from build123d import *

# Parameters (mm, degrees)
SKETCH2_R           = 19
SKETCH2_R_2         = 1.3
BOSS_EXTRUDE1_DEPTH = 8
SKETCH3_R           = 30
SKETCH3_R_2         = 17.487995661
BOSS_EXTRUDE2_DEPTH = 8
SKETCH4_R           = 2.9
BOSS_EXTRUDE3_DEPTH = 2
SKETCH6_R           = 5
BOSS_EXTRUDE4_DEPTH = 3
SKETCH5_R           = 3
CUT_EXTRUDE1_DEPTH  = 3
SKETCH7_R           = 25
CUT_EXTRUDE2_DEPTH  = 8
FILLET2_R           = 5


with BuildPart() as part:
    # Sketch2 → Boss-Extrude1 (new body)
    with BuildSketch(Plane.XY.offset(10)):
        Circle(SKETCH2_R)
        with Locations((0, -2.215732779)):
            Circle(SKETCH2_R_2, mode=Mode.SUBTRACT)
        with Locations((3.9, -2.215732779)):
            Circle(SKETCH2_R_2, mode=Mode.SUBTRACT)
        with Locations((7.8, -2.215732779)):
            Circle(SKETCH2_R_2, mode=Mode.SUBTRACT)
        with Locations((11.7, -2.215732779)):
            Circle(SKETCH2_R_2, mode=Mode.SUBTRACT)
        with Locations((1.95, -5.593231854)):
            Circle(SKETCH2_R_2, mode=Mode.SUBTRACT)
        with Locations((3.9, -8.970730929)):
            Circle(SKETCH2_R_2, mode=Mode.SUBTRACT)
        with Locations((5.850000003, -12.348230002)):
            Circle(SKETCH2_R_2, mode=Mode.SUBTRACT)
        with Locations((-1.95, -5.593231854)):
            Circle(SKETCH2_R_2, mode=Mode.SUBTRACT)
        with Locations((-3.9, -8.970730929)):
            Circle(SKETCH2_R_2, mode=Mode.SUBTRACT)
        with Locations((-5.85, -12.348230004)):
            Circle(SKETCH2_R_2, mode=Mode.SUBTRACT)
        with Locations((-3.9, -2.215732779)):
            Circle(SKETCH2_R_2, mode=Mode.SUBTRACT)
        with Locations((-7.8, -2.215732779)):
            Circle(SKETCH2_R_2, mode=Mode.SUBTRACT)
        with Locations((-11.7, -2.215732779)):
            Circle(SKETCH2_R_2, mode=Mode.SUBTRACT)
        with Locations((-1.950000001, 1.161766295)):
            Circle(SKETCH2_R_2, mode=Mode.SUBTRACT)
        with Locations((-3.9, 4.53926537)):
            Circle(SKETCH2_R_2, mode=Mode.SUBTRACT)
        with Locations((-5.85, 7.916764445)):
            Circle(SKETCH2_R_2, mode=Mode.SUBTRACT)
        with Locations((-7.8, 11.29426352)):
            Circle(SKETCH2_R_2, mode=Mode.SUBTRACT)
        with Locations((1.95, 1.161766295)):
            Circle(SKETCH2_R_2, mode=Mode.SUBTRACT)
        with Locations((3.9, 4.53926537)):
            Circle(SKETCH2_R_2, mode=Mode.SUBTRACT)
        with Locations((5.85, 7.916764445)):
            Circle(SKETCH2_R_2, mode=Mode.SUBTRACT)
        with Locations((7.8, 11.29426352)):
            Circle(SKETCH2_R_2, mode=Mode.SUBTRACT)
        with Locations((5.85, 1.161766295)):
            Circle(SKETCH2_R_2, mode=Mode.SUBTRACT)
        with Locations((7.8, 4.53926537)):
            Circle(SKETCH2_R_2, mode=Mode.SUBTRACT)
        with Locations((9.75, 1.161766295)):
            Circle(SKETCH2_R_2, mode=Mode.SUBTRACT)
        with Locations((11.7, 4.53926537)):
            Circle(SKETCH2_R_2, mode=Mode.SUBTRACT)
        with Locations((9.749099848, 7.918323553)):
            Circle(SKETCH2_R_2, mode=Mode.SUBTRACT)
        with Locations((13.650900152, 1.160207187)):
            Circle(SKETCH2_R_2, mode=Mode.SUBTRACT)
        with Locations((5.850000208, -5.594790783)):
            Circle(SKETCH2_R_2, mode=Mode.SUBTRACT)
        with Locations((9.750000208, -5.594790782)):
            Circle(SKETCH2_R_2, mode=Mode.SUBTRACT)
        with Locations((7.800000209, -8.972289857)):
            Circle(SKETCH2_R_2, mode=Mode.SUBTRACT)
        with Locations((-0.00134976, -8.973069502)):
            Circle(SKETCH2_R_2, mode=Mode.SUBTRACT)
        with Locations((1.94865024, -12.350568576)):
            Circle(SKETCH2_R_2, mode=Mode.SUBTRACT)
        with Locations((-1.95134976, -12.350568576)):
            Circle(SKETCH2_R_2, mode=Mode.SUBTRACT)
        with Locations((-5.852699936, -5.594791143)):
            Circle(SKETCH2_R_2, mode=Mode.SUBTRACT)
        with Locations((-7.802699936, -8.972290217)):
            Circle(SKETCH2_R_2, mode=Mode.SUBTRACT)
        with Locations((-9.752699936, -5.594791143)):
            Circle(SKETCH2_R_2, mode=Mode.SUBTRACT)
        with Locations((-5.852700144, 1.161765936)):
            Circle(SKETCH2_R_2, mode=Mode.SUBTRACT)
        with Locations((-9.752700144, 1.161765936)):
            Circle(SKETCH2_R_2, mode=Mode.SUBTRACT)
        with Locations((-7.802700144, 4.53926501)):
            Circle(SKETCH2_R_2, mode=Mode.SUBTRACT)
        with Locations((-11.702700144, 4.53926501)):
            Circle(SKETCH2_R_2, mode=Mode.SUBTRACT)
        with Locations((-9.751799992, 7.918323194)):
            Circle(SKETCH2_R_2, mode=Mode.SUBTRACT)
        with Locations((-13.653600295, 1.160206827)):
            Circle(SKETCH2_R_2, mode=Mode.SUBTRACT)
        with Locations((-0.001350176, 4.540044654)):
            Circle(SKETCH2_R_2, mode=Mode.SUBTRACT)
        with Locations((-1.951350176, 7.917543729)):
            Circle(SKETCH2_R_2, mode=Mode.SUBTRACT)
        with Locations((1.948649824, 7.917543729)):
            Circle(SKETCH2_R_2, mode=Mode.SUBTRACT)
        with Locations((-0.001350176, 11.295042804)):
            Circle(SKETCH2_R_2, mode=Mode.SUBTRACT)
        with Locations((3.900450128, 11.295042804)):
            Circle(SKETCH2_R_2, mode=Mode.SUBTRACT)
        with Locations((-3.903150479, 11.295042804)):
            Circle(SKETCH2_R_2, mode=Mode.SUBTRACT)
    extrude(amount=BOSS_EXTRUDE1_DEPTH)

    # Sketch3 → Boss-Extrude2 (add)
    with BuildSketch(Plane.XY.offset(18)):
        Circle(SKETCH3_R)
        Circle(SKETCH3_R_2, mode=Mode.SUBTRACT)
    extrude(amount=-BOSS_EXTRUDE2_DEPTH)

    # Sketch4 → Boss-Extrude3 (add)
    with BuildSketch(Plane.XY.offset(18)):
        with Locations((0, 25)):
            Circle(SKETCH4_R)
        with Locations((21.650635095, -12.5)):
            Circle(SKETCH4_R)
        with Locations((-21.650635095, -12.5)):
            Circle(SKETCH4_R)
    extrude(amount=BOSS_EXTRUDE3_DEPTH)

    # Sketch6 → Boss-Extrude4 (add)
    with BuildSketch(Plane(origin=(0, 0, 10), x_dir=(-1, 0, 0), z_dir=(0, 0, -1))):
        with Locations((0, 30)):
            Circle(SKETCH6_R)
        with Locations((25.980762114, -15)):
            Circle(SKETCH6_R)
        with Locations((-25.980762114, -15)):
            Circle(SKETCH6_R)
    extrude(amount=-BOSS_EXTRUDE4_DEPTH)

    # Sketch5 → Cut-Extrude1 (cut)
    with BuildSketch(Plane(origin=(0, 0, 10), x_dir=(-1, 0, 0), z_dir=(0, 0, -1))):
        with Locations((0, 25)):
            Circle(SKETCH5_R)
        with Locations((21.650635095, -12.5)):
            Circle(SKETCH5_R)
        with Locations((-21.650635095, -12.5)):
            Circle(SKETCH5_R)
    extrude(amount=-CUT_EXTRUDE1_DEPTH, mode=Mode.SUBTRACT)

    # Sketch7 → Cut-Extrude2 (cut)
    with BuildSketch(Plane(origin=(0, 0, 10), x_dir=(-1, 0, 0), z_dir=(0, 0, -1))):
        with Locations((36.373066959, 21)):
            Circle(SKETCH7_R)
        with Locations((0, -42)):
            Circle(SKETCH7_R)
        with Locations((-36.373066959, 21)):
            Circle(SKETCH7_R)
    extrude(amount=-CUT_EXTRUDE2_DEPTH, mode=Mode.SUBTRACT)

    # Fillet2
    fillet2_edges = [part.edges().sort_by_distance(p)[0] for p in [
        (29.836243213, -3.130270104, 14),
        (12.207228175, 27.404079628, 14),
        (-12.207228175, 27.404079628, 14),
        (-29.836243213, -3.130270104, 14),
        (-17.629015038, -24.273809524, 14),
        (17.629015038, -24.273809524, 14),
    ]]
    fillet(fillet2_edges, radius=FILLET2_R)


solid = part.part
Can you work these out from the model? Positions are in its coordinate system, mm. A direction names the side the tool comes from. Give positions to 0.01 mm unless a question says otherwise; leave off trailing zeros. Write each question's results on one line, items separated by ' | '.
1) I'm going to push flat-ended pins straight in: pin 1 Ø2 at (x, z) = (0.5, 13) entering from -Y; pin 2 Ø6 at (x, z) = (-2, 19) entering from +Y; pin 3 Ø4 at (x, y) = (-5.85, 7.92) entering from +Z; pin 4 Ø4 at (x, y) = (1.95, -5.59) entering from -Z. Where does each tip first touch, or does it pass through?
Final values:
pin 1: stops at y = -17.05 | pin 2: stops at y = 30 | pin 3: stops at z = 18 | pin 4: stops at z = 10
2) If we mould it in two halves opening along X, with no side actions, what happens to faces 1 (the face through (4.818, 7.126, 13.944)), 2 (the face through (0, 32, 13))? For each: pulls with the +X half, pulls with the -X half, needs draft (parallel to the pull), parting line crosses it, or undercut.
Final values:
face 1: undercut | face 2: needs draft
3) On a 3-axis mill with a long thin cutter (end or side, diameter ignored), from which of +Z, -Z, +X, -X, +Y, -Y can I reach the whole of each face in a straight line? I mean faces 3 (the face through (-4.072, 12.584, 13.944)), 4 (the face through (24.33, -13.61, 18.99)), 5 (the face through (18.88, -13.65, 11.48)). Say none if no direction works.
Final values:
face 3: +Z, -Z | face 4: +Z | face 5: -Z
4) Suppose I cut it at A-A, the plane z = 13.75. Give the number of separate pieces and of enclosed holes in the cut face, then the cut area to 3 significant figures.
Final values:
separate pieces: 1 | enclosed holes: 48 | area: 1,610 mm^2
5) Please list where these lines run through material, in increasing order: line 1 along Y through (x, z) = (7.8, 14.5); line 2 along Y through (x, z) = (6, 12); line 3 along X through (y, z) = (-8, 10.75). Write a range as [from, to].
Final values:
line 1: y = [-18.25, -10.27], [-7.67, -3.52], [-0.92, 3.24], [5.84, 9.99], [12.59, 28.97] | line 2: y = [-17.73, -13.64], [-11.06, -6.89], [-4.3, -0.13], [2.45, 6.63], [9.21, 29.39] | line 3: x = [-28.91, -8.67], [-6.94, -4.76], [-3.04, -0.86], [0.86, 3.04], [4.76, 6.94], [8.66, 28.91]
